Can you work these out from the model? Positions are in its coordinate system, mm. A direction names the side the tool comes from. Coordinates: 2 decimals unless noted, no trailing zeros. Order: outer loops, then holes, each group sorted by start corner. A loop starts at its lowest first (then second) coordinate and runs counter-clockwise, first axis right, second up. Notation, with made-up numbers: (3.25, 62.25) -> (8.25, 62.25) arc R19 ccw to (8.25, 94.25) -> close; hole circle Ø5 at (83, 39.25). An arc over 180 degrees is marked (long way). Answer in a Markdown table with one row per item. Add a question column.
1. Imagine slicing it at B-B on x = 27. Write out the boundary of the cut face in (y, z), plus the area to 3 significant figures.
2. Will these pins go through, and if not, where does the flat tip stop? pin 1 (0.6 mm diameter, centred on x = 56.5, y = 18, fed in from -Z); pin 2 (2 mm diameter, centred on y = -7, z = -27.5, fed in from +X); pin 3 (10 mm diameter, centred on y = -2.5, z = -41, fed in from +X).
3. On a 3-axis mill with a long thin cutter (end or side, diameter ignored), from which of +Z, -Z, +X, -X, +Y, -Y can I reach the whole of each face in a straight line? I mean faces 4 (the face through (29, 16, -23)), 5 (the face through (94, 18, 7)), 6 (the face through (9, 0, -11)). Say none if no direction works.
4. Imagine slicing it at A-A on y = 14. Write out the boundary of the cut face in (x, z), plus the area to 3 significant figures.
5. We'd pull the mould along Z, two halves only. Please class faces 1 (the face through (22, 0, 10)), 2 (the face through (73, -18, 2)), 3 (the face through (22, 0, -12)): pulls with the +Z half, pulls with the -Z half, needs draft (parallel to the pull), parting line crosses it, or undercut.
6. If I drill on line 1 along Z through (x, y) = (80, 16.75); line 2 along Z through (x, y) = (13, -15.5); line 3 along Z through (x, y) = (80, -13), over which ranges is the centre line in solid material (lowest first)? Write a range as [from, to].
7. Imagine slicing it at C-C on x = 65.5. Write out the boundary of the cut face in (y, z), plus the area to 3 significant figures.
8. Imagine slicing it at D-D on x = 8. Write out the boundary of the cut face in (y, z).
from build123d import *

# Parameters (mm, degrees)
F1_DEPTH  = 16
F2_W      = 70
F2_H      = 3
F3_DEPTH  = 2
F4_W      = 50
F4_H      = 14
F5_DEPTH  = 2
F6_R      = 1
F9_DEPTH  = 32.3
F11_DEPTH = 38.001
F13_D     = 4
F14_R     = 3
F14_R_2   = 2
F15_DEPTH = 5
F16_R     = 3


# Not quite as in the source:
# - ends of sketch curves that miss each other by under 0.0002 mm in the source are joined
# - a pattern or mirror of a feature is missing from the dataset's text; its kind, count and spacing are read off the source's solid


with BuildPart() as f1:
    # F0 (on Front) → F1 (new body)
    with BuildSketch(Plane.XZ):
        with BuildLine():
            Line((94, 10.9999997337), (0, 10.9999997337))
            ThreePointArc((0, 10.9999997337), (-10.9999997337, 0), (0, -10.9999997337))
            Line((0, -10.9999997337), (19, -10.9999997337))
            ThreePointArc((19, -10.9999997337), (21.9703860558, -11.9779596195), (23.7788047483, -14.5292770618))
            ThreePointArc((23.7788047483, -14.5292770618), (48.7042113744, -47.9191442908), (89.135710582, -57.9915323328))
            ThreePointArc((89.135710582, -57.9915323328), (95.6273356348, -58.9810862831), (100.9536755577, -62.8217263174))
            Line((100.9536755577, -62.8217263174), (102.4712510554, -61.5190536469))
            ThreePointArc((102.4712510554, -61.5190536469), (96.3776978188, -57.1271725396), (88.9514269277, -56))
            ThreePointArc((88.9514269277, -56), (49.8169100213, -46.2572353593), (25.6903263931, -13.9409880714))
            ThreePointArc((25.6903263931, -13.9409880714), (23.1585403199, -10.3691437881), (19, -9))
            Line((19, -9), (0, -9))
            ThreePointArc((0, -9), (-9, 0), (0, 9))
            Line((0, 9), (94, 9))
            Line((94, 9), (94, 10.9999997337))
        make_face()
    extrude(amount=F1_DEPTH)

    # F2 (on face) → F3 (join)
    with BuildSketch(Plane.XY.offset(10.9999997337)):
        with Locations((59, -17.5)):
            Rectangle(F2_W, F2_H)
    extrude(amount=-F3_DEPTH)

    # F4 (on face) → F5 (join)
    with BuildSketch(Plane.XZ.offset(19)):
        with Locations((69, 3.9999997337)):
            Rectangle(F4_W, F4_H)
    extrude(amount=-F5_DEPTH)

    # F6
    f6_edges = [f1.edges().sort_by_distance(p)[0] for p in [
        (59, -19, 11),
    ]]
    fillet(f6_edges, radius=F6_R)

    # F7: F1 across plane


with BuildPart() as f1_1:
    add(f1.part)
    add(f1.part.mirror(Plane.XZ))

    # F8 (on Top) → F9 (cut)
    with BuildSketch(Plane.XY):
        with BuildLine():
            Line((94, 12), (34, 12))
            ThreePointArc((34, 12), (22, 0), (34, -12))
            Line((34, -12), (94, -12))
            Line((94, -12), (94, 12))
        make_face()
    extrude(amount=F9_DEPTH, mode=Mode.SUBTRACT)

    # F10 (on face) → F11 (cut, through all)
    with BuildSketch(Plane.XZ.offset(19)):
        with BuildLine():
            ThreePointArc((50, 4.9999997337), (47, 1.9999997337), (50, -1.0000002663))
            Line((50, -1.0000002663), (70, -1.0000002663))
            ThreePointArc((70, -1.0000002663), (73, 1.9999997337), (70, 4.9999997337))
            Line((70, 4.9999997337), (50, 4.9999997337))
        make_face()
    extrude(amount=-F11_DEPTH, mode=Mode.SUBTRACT)

    # F13 (through all)
    with Locations(Plane.XZ.offset(19)):
        with Locations((80, 2.9999997337)):
            Hole(F13_D / 2)

    # F14 (on face) → F15 (join)
    with BuildSketch(Plane(origin=(0, -17, 0), x_dir=(-1, 0, 0), z_dir=(0, 1, 0))):
        with Locations((-80, 2.9999997337)):
            Circle(F14_R)
        with Locations((-80, 2.9999997337)):
            Circle(F14_R_2, mode=Mode.SUBTRACT)
    f15 = extrude(amount=F15_DEPTH)

    # F15_copies: F15 across plane
    add(f15.mirror(Plane.ZX))

    # F16
    f16_edges = [f1_1.edges().sort_by_distance(p)[0] for p in [
        (94, -18, -3),
        (94, 18, -3),
        (44, -18, -3),
        (44, 18, -3),
    ]]
    fillet(f16_edges, radius=F16_R)


solid = f1_1.part
Answers follow:
| question | item | result |
|---|---|---|
| 1 | outline | (-19, 9) -> (-9.75, 9) -> (-9.75, 11) -> (-18, 11) arc R1 ccw to (-19, 10) -> close; (-16, -22.82) -> (16, -22.82) -> (16, -17.74) -> (-16, -17.74) -> close; (9.75, 9) -> (19, 9) -> (19, 10) arc R1 ccw to (18, 11) -> (9.75, 11) -> close |
| 1 | area | 199 mm² |
| 2 | pin 1 | stops at z = -3 |
| 2 | pin 2 | stops at x = 32.41 |
| 2 | pin 3 | stops at x = 49.43 |
| 3 | face 4 | -Z, -X, +Y |
| 3 | face 5 | +Z, +X, +Y, -Y |
| 3 | face 6 | -Z, -X, +Y, -Y |
| 4 | outline | (0, -11) -> (19, -11) arc R5 cw to (23.78, -14.53) arc R62 ccw to (89.14, -57.99) arc R14 cw to (100.95, -62.82) -> (102.47, -61.52) arc R16 ccw to (88.95, -56) arc R60 cw to (25.69, -13.94) arc R7 ccw to (19, -9) -> (0, -9) arc R9 cw to (0, 9) -> (94, 9) -> (94, 11) -> (0, 11) arc R11 ccw to start; circle Ø6 at (80, 3); hole circle Ø4 at (80, 3) |
| 4 | area | 515 mm² |
| 5 | face 1 | needs draft |
| 5 | face 2 | undercut |
| 5 | face 3 | pulls with the -Z half |
| 6 | line 1 | z = [0, 1], [5, 6], [9, 11] |
| 6 | line 2 | z = [-11, -9], [9, 11] |
| 6 | line 3 | z = [-58.22, -56.22], [0, 1], [5, 6], [9, 11] |
| 7 | outline | (-19, -3) -> (-17, -3) -> (-17, -1) -> (-19, -1) -> close; (-19, 5) -> (-17, 5) -> (-17, 9) -> (-12, 9) -> (-12, 11) -> (-18, 11) arc R1 ccw to (-19, 10) -> close; (-16, -55.76) -> (16, -55.76) -> (16, -53.67) -> (-16, -53.67) -> close; (12, 9) -> (17, 9) -> (17, 5) -> (19, 5) -> (19, 10) arc R1 ccw to (18, 11) -> (12, 11) -> close; (17, -3) -> (19, -3) -> (19, -1) -> (17, -1) -> close |
| 7 | area | 118 mm² |
| 8 | outline | (-16, -11) -> (16, -11) -> (16, -9) -> (-16, -9) -> close; (-16, 9) -> (16, 9) -> (16, 11) -> (-16, 11) -> close |
